```python
from build123d import *

# Parameters (mm, degrees)
F0_R     = 1.651
F0_W     = 6.35
F0_H     = 31.75
F0_R_2   = 1.905
F1_DEPTH = 1.5875
F2_W     = 12.7
F2_H     = 41.91
F2_W_2   = 13.97
F3_DEPTH = 6.35
F4_R     = 2.921
F4_R_2   = 1.016
F5_DEPTH = 6.35
F6_DEPTH = 6.35


with BuildPart() as f1:
    # F0 (on Top) → F1 (new body)
    with BuildSketch(Plane.XY):
        with BuildLine():
            Line((42.545, -28.067), (42.545, 28.067))
            Line((42.545, 28.067), (-36.195, 28.067))
            ThreePointArc((-36.195, 28.067), (-40.6851280605, 26.2071280605), (-42.545, 21.717))
            Line((-42.545, 21.717), (-42.545, -28.067))
            Line((-42.545, -28.067), (-29.845, -28.067))
            Line((-29.845, -28.067), (42.545, -28.067))
        make_face()
        with BuildLine():
            Line((48.895, 28.067), (42.545, 28.067))
            Line((42.545, 28.067), (42.545, -28.067))
            Line((42.545, -28.067), (48.895, -28.067))
            ThreePointArc((48.895, -28.067), (53.3851280605, -26.2071280605), (55.245, -21.717))
            Line((55.245, -21.717), (55.245, 21.717))
            ThreePointArc((55.245, 21.717), (53.3851280605, 26.2071280605), (48.895, 28.067))
        make_face()
        with Locations((48.895, -21.717)):
            Circle(F0_R, mode=Mode.SUBTRACT)
        with Locations((48.895, 0.762)):
            Rectangle(F0_W, F0_H, mode=Mode.SUBTRACT)
        with Locations((48.895, 23.241)):
            Circle(F0_R, mode=Mode.SUBTRACT)
        with BuildLine():
            Line((-29.845, -34.417), (-29.845, -28.067))
            Line((-29.845, -28.067), (-42.545, -28.067))
            Line((-42.545, -28.067), (-42.545, -34.417))
            ThreePointArc((-42.545, -34.417), (-40.6851280605, -38.9071280605), (-36.195, -40.767))
            ThreePointArc((-36.195, -40.767), (-31.7048719395, -38.9071280605), (-29.845, -34.417))
        make_face()
        with Locations((-36.195, -34.417)):
            Circle(F0_R_2, mode=Mode.SUBTRACT)
    extrude(amount=F1_DEPTH)

    # F2 (on face) → F3 (cut)
    with BuildSketch(Plane.XY.offset(1.5875)):
        with Locations((30.48, 0)):
            Rectangle(F2_W, F2_H)
        with Locations((10.795, 0)):
            Rectangle(F2_W_2, F2_H)
        with Locations((-9.525, 0)):
            Rectangle(F2_W_2, F2_H)
        with Locations((-29.845, 0)):
            Rectangle(F2_W_2, F2_H)
    extrude(amount=-F3_DEPTH, mode=Mode.SUBTRACT)

    # F4 (on face) → F5 (join)
    with BuildSketch(Plane.XY.offset(1.5875)):
        with Locations((38.989, 24.511)):
            Circle(F4_R)
        with Locations((38.989, 24.511)):
            Circle(F4_R_2, mode=Mode.SUBTRACT)
        with Locations((38.989, -24.511)):
            Circle(F4_R)
        with Locations((38.989, -24.511)):
            Circle(F4_R_2, mode=Mode.SUBTRACT)
        with Locations((-19.177, 24.511)):
            Circle(F4_R)
        with Locations((-19.177, 24.511)):
            Circle(F4_R_2, mode=Mode.SUBTRACT)
        with Locations((-19.177, -24.511)):
            Circle(F4_R)
        with Locations((-19.177, -24.511)):
            Circle(F4_R_2, mode=Mode.SUBTRACT)
    extrude(amount=F5_DEPTH)

    # F4 (on face) → F6 (cut)
    with BuildSketch(Plane.XY.offset(1.5875)):
        with Locations((38.989, -24.511)):
            Circle(F4_R_2)
        with Locations((-19.177, 24.511)):
            Circle(F4_R_2)
        with Locations((38.989, 24.511)):
            Circle(F4_R_2)
        with Locations((-19.177, -24.511)):
            Circle(F4_R_2)
    extrude(amount=-F6_DEPTH, mode=Mode.SUBTRACT)


solid = f1.part
```
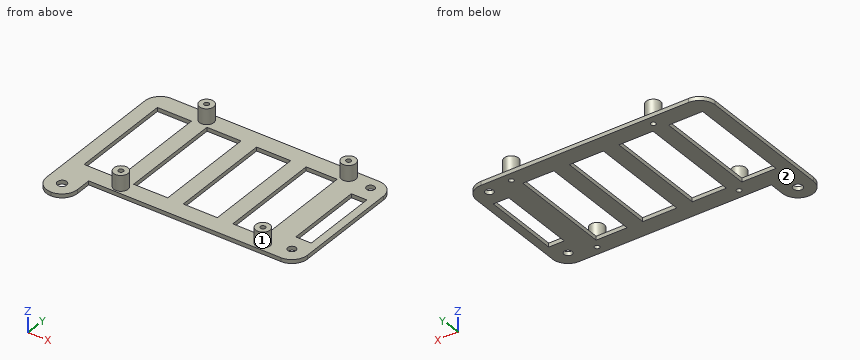
Check sheet for the modelled part. Datum: model origin and axes. Units: mm. Face numbers are marked on the shaded views. Coordinates: 2 decimals unless noted, no trailing zeros. Loops run counter-clockwise (first coordinate to the right, second up) from the corner with the lowest first, then second, coordinate; pieces in that order, holes last.
1) Sectioned sample at A-A (x = -8). Record the boundary of the cut face in (y, z) (1 decimal), and give its area (3 significant figures).
2) Sectioned sample at C-C (z = 3.25). Record the boundary of the cut face in (x, y) (3 decimals), and give its area (3 significant figures).
3) Sectioned sample at D-D (y = -17.5). Record the boundary of the cut face in (x, z) (1 decimal), and give its area (3 significant figures).
4) Sectioned sample at B-B (y = 13). Record the boundary of the cut face in (x, z) (1 decimal), and give its area (3 significant figures).
5) Material ranges on probe 1 along X at (y, z) = (-0.5, 0.5) (3 decimals); probe 2 along Z at (x, y) = (30, 22); probe 3 along X at (y, z) = (22, 7), recorded low to high.
6) Gauge pin test, flat ends, axial feed: pin 1 (1.7 mm diameter, centred on x = -27.5, z = 1, fed in from -Y); pin 2 (5.5 mm diameter, centred on x = 48.895, y = -21.717, fed in from +Z); pin 3 (0.8 mm diameter, centred on x = 49.5, z = 1, fed in from +Y); pin 4 (3 mm diameter, centred on y = 19.5, z = 3, fed in from +X) (3 decimals). Record the tip position at first contact, or that the pin passes through.
7) Release check for a two-part mould opening along Y. For the marked faces 1 and 2 record: released by +Y, released by -Y, zero draft, split by the parting line, or undercut.
Check sheet entries:
1. outline: (-28.1, 0) - (-21, 0) - (-21, 1.6) - (-28.1, 1.6) - close; (21, 0) - (28.1, 0) - (28.1, 1.6) - (21, 1.6) - close
1. area: 22.6 mm2
2. outline: circle Ø5.842 at (-19.177, -24.511); circle Ø5.842 at (-19.177, 24.511); circle Ø5.842 at (38.989, -24.511); circle Ø5.842 at (38.989, 24.511); hole circle Ø2.032 at (-19.177, -24.511); hole circle Ø2.032 at (-19.177, 24.511); hole circle Ø2.032 at (38.989, -24.511); hole circle Ø2.032 at (38.989, 24.511)
2. area: 94.2 mm2
3. outline: (-42.5, 0) - (-36.8, 0) - (-36.8, 1.6) - (-42.5, 1.6) - close; (-22.9, 0) - (-16.5, 0) - (-16.5, 1.6) - (-22.9, 1.6) - close; (-2.5, 0) - (3.8, 0) - (3.8, 1.6) - (-2.5, 1.6) - close; (17.8, 0) - (24.1, 0) - (24.1, 1.6) - (17.8, 1.6) - close; (36.8, 0) - (55.2, 0) - (55.2, 1.6) - (36.8, 1.6) - close
3. area: 68.5 mm2
4. outline: (-42.5, 0) - (-36.8, 0) - (-36.8, 1.6) - (-42.5, 1.6) - close; (-22.9, 0) - (-16.5, 0) - (-16.5, 1.6) - (-22.9, 1.6) - close; (-2.5, 0) - (3.8, 0) - (3.8, 1.6) - (-2.5, 1.6) - close; (17.8, 0) - (24.1, 0) - (24.1, 1.6) - (17.8, 1.6) - close; (36.8, 0) - (45.7, 0) - (45.7, 1.6) - (36.8, 1.6) - close; (52.1, 0) - (55.2, 0) - (55.2, 1.6) - (52.1, 1.6) - close
4. area: 58.5 mm2
5. probe 1: x = -42.545 to -36.83, -22.86 to -16.51, -2.54 to 3.81, 17.78 to 24.13, 36.83 to 45.72, 52.07 to 55.245
5. probe 2: z = 0 to 1.59
5. probe 3: x = -20.67 to -17.68, 37.5 to 40.48
6. pin 1: stops at y = -28.07
6. pin 2: stops at z = 1.59
6. pin 3: stops at y = 28.06
6. pin 4: stops at x = 55.245
7. face 1: undercut
7. face 2: zero draft
